Input: part model. Units: mm. Frame: model coordinates. A direction names the side the tool comes from. Coordinates: 2 decimals unless noted, no trailing zeros. Loops run counter-clockwise (first coordinate to the right, second up) from the corner with the lowest first, then second, coordinate; pieces in that order, holes last.
Item 1: Reachability of faces 1 (the flat face through (155, -25, -188)), 2 (the flat face through (-125, -41, -175)), 3 (the flat face through (-95, -25, 187)) from +Z, -Z, +X, -X, +Y, -Y: full face, straight path, thin tool, end or side. Return the list, or none.
Item 2: Section C-C on y = 305. Return loops of the section in (x, z), and give its area (3 significant figures).
Item 3: Pull-direction query (Z, two-part tool) for faces 4 (the flat face through (-3, 83, 200)), 5 (the flat face through (-88, 178, -15)), 6 (the cylindrical face through (139.985, -24.34, -187.675)); classes: released by +Z, released by -Z, zero draft, split by the parting line, or undercut.
Item 4: Section B-B on y = 136.5. Return loops of the section in (x, z).
Item 5: Section D-D on x = 125. Return loops of the section in (y, z).
Item 6: Ray query, line 1 along Z through (x, y) = (-39.5, 155.5); line 2 along X through (y, z) = (158, -143); line 3 along Y through (x, z) = (125, 191). Return the intervals inside material, ascending.
Item 7: Section A-A on z = 0. Return loops of the section in (x, y).
Item 8: Contact query for flat-ended pins moving along their axis: P1, Ø1, axis at x = 151.5, z = -36, coming from the -Y side; P2, Ø23, axis at y = 305, z = 0, coming from the +X side; P3, Ø24, axis at x = -125, y = -25, coming from the +Z side; P4, Ø20, axis at y = -16.5, z = -190.5, coming from the -X side. Output: stop coordinate, or through.
```python
from build123d import *

# Parameters (mm, degrees)
SKETCH1_W            = 450
SKETCH1_H            = 400
BOSS_EXTRUDE1_DEPTH  = 220
SKETCH2_W            = 425
SKETCH2_H            = 375
CUT_EXTRUDE1_DEPTH   = 160
SKETCH3_W            = 280
SKETCH3_H            = 140
CUT_EXTRUDE2_DEPTH   = 12.5
SKETCH4_W            = 30
SKETCH4_H            = 30
BOSS_EXTRUDE2_DEPTH  = 260
SKETCH5_R            = 10
CUT_EXTRUDE3_DEPTH   = 30
SKETCH6_W            = 60
SKETCH6_H            = 25
BOSS_EXTRUDE3_DEPTH  = 50
SKETCH7_R            = 15
CUT_EXTRUDE4_DEPTH   = 25
CUT_EXTRUDE5_START   = -25
SKETCH8_R            = 15
CUT_EXTRUDE5_DEPTH   = 25
CUT_EXTRUDE6_START   = -187.5
CUT_EXTRUDE6_DEPTH   = 375
CUT_EXTRUDE6_2_DEPTH = 172.5
CUT_EXTRUDE6_START_2 = 15
CUT_EXTRUDE6_3_DEPTH = 172.5
SKETCH10_W           = 375
SKETCH10_H           = 197.182681999
CUT_EXTRUDE7_DEPTH   = 12.5


# Read off the part's stored shape, not the designer's step: Cut-Extrude6
with BuildPart() as part:
    # Sketch1 → Boss-Extrude1 (new body)
    with BuildSketch(Plane(origin=(0, 0, 0), x_dir=(1, 0, 0), z_dir=(0, 1, 0))):
        Rectangle(SKETCH1_W, SKETCH1_H)
    extrude(amount=BOSS_EXTRUDE1_DEPTH)

    # Sketch2 → Cut-Extrude1 (cut)
    with BuildSketch(Plane(origin=(0, 220, 0), x_dir=(1, 0, 0), z_dir=(0, 1, 0))):
        Rectangle(SKETCH2_W, SKETCH2_H)
    extrude(amount=-CUT_EXTRUDE1_DEPTH, mode=Mode.SUBTRACT)

    # Sketch3 → Cut-Extrude2 (cut)
    with BuildSketch(Plane(origin=(225, 0, 0), x_dir=(0, 0, -1), z_dir=(1, 0, 0))):
        with Locations((0, 150)):
            Rectangle(SKETCH3_W, SKETCH3_H)
    extrude(amount=-CUT_EXTRUDE2_DEPTH, mode=Mode.SUBTRACT)

    # Sketch4 → Boss-Extrude2 (add)
    with BuildSketch(Plane(origin=(0, 60, 0), x_dir=(1, 0, 0), z_dir=(0, 1, 0))):
        with Locations((-87.5, 0)):
            Rectangle(SKETCH4_W, SKETCH4_H)
    extrude(amount=BOSS_EXTRUDE2_DEPTH)

    # Sketch5 → Cut-Extrude3 (cut)
    with BuildSketch(Plane(origin=(-72.5, 0, 0), x_dir=(0, 0, -1), z_dir=(1, 0, 0))):
        with Locations((0, 305)):
            Circle(SKETCH5_R)
    extrude(amount=-CUT_EXTRUDE3_DEPTH, mode=Mode.SUBTRACT)

    # Sketch6 → Boss-Extrude3 (add)
    with BuildSketch(Plane.XZ):
        with Locations((125, 187.5)):
            Rectangle(SKETCH6_W, SKETCH6_H)
        with Locations((-125, 187.5)):
            Rectangle(SKETCH6_W, SKETCH6_H)
        with Locations((-125, -187.5)):
            Rectangle(SKETCH6_W, SKETCH6_H)
        with Locations((125, -187.5)):
            Rectangle(SKETCH6_W, SKETCH6_H)
    extrude(amount=BOSS_EXTRUDE3_DEPTH)

    # Sketch7 → Cut-Extrude4 (cut)
    with BuildSketch(Plane(origin=(0, 0, -200), x_dir=(-1, 0, 0), z_dir=(0, 0, -1))):
        with Locations((125, -25)):
            Circle(SKETCH7_R)
        with Locations((-125, -25)):
            Circle(SKETCH7_R)
    extrude(amount=-CUT_EXTRUDE4_DEPTH, mode=Mode.SUBTRACT)

    # Sketch8 → Cut-Extrude5 (cut)
    with BuildSketch(Plane.XY.offset(200).offset(CUT_EXTRUDE5_START)):
        with Locations(Location((-125, -25, 0), (0, 0, 180))):
            Circle(SKETCH8_R)
        with Locations(Location((125, -25, 0), (0, 0, 180))):
            Circle(SKETCH8_R)
    extrude(amount=CUT_EXTRUDE5_DEPTH, mode=Mode.SUBTRACT)

    # Cut-Extrude6 outline → Cut-Extrude6 (cut)
    with BuildSketch(Plane.XY.offset(CUT_EXTRUDE6_START)):
        Polygon((-102.5, 60), (-212.5, 60), (-212.5, 22.817318001), (-102.5, 32.441070989), align=None)
        Polygon((212.5, 60), (-72.5, 60), (-72.5, 35.065730895), align=None)
    extrude(amount=CUT_EXTRUDE6_DEPTH, mode=Mode.SUBTRACT)

    # Cut-Extrude6 2 outline → Cut-Extrude6 2 (cut)
    with BuildSketch(Plane.XY.offset(CUT_EXTRUDE6_START)):
        Polygon((-72.5, 60), (-102.5, 60), (-102.5, 32.441070989), (-72.5, 35.065730895), align=None)
    extrude(amount=CUT_EXTRUDE6_2_DEPTH, mode=Mode.SUBTRACT)

    # Cut-Extrude6 3 outline → Cut-Extrude6 3 (cut)
    with BuildSketch(Plane.XY.offset(CUT_EXTRUDE6_START_2)):
        Polygon((-72.5, 60), (-102.5, 60), (-102.5, 32.441070989), (-72.5, 35.065730895), align=None)
    extrude(amount=CUT_EXTRUDE6_3_DEPTH, mode=Mode.SUBTRACT)

    # Sketch10 → Cut-Extrude7 (cut)
    with BuildSketch(Plane(origin=(-212.5, 0, 0), x_dir=(0, 0, -1), z_dir=(1, 0, 0))):
        with Locations((0, 121.408659)):
            Rectangle(SKETCH10_W, SKETCH10_H)
    extrude(amount=-CUT_EXTRUDE7_DEPTH, mode=Mode.SUBTRACT)


solid = part.part
```
Results found:
1. face 1: +Z, -Z, +X, -Y
1. face 2: +X, -X, -Y
1. face 3: +Z, -Z, -Y
2. outline: (-102.5, -15) - (-72.5, -15) - (-72.5, -10) - (-102.5, -10) - close; (-102.5, 10) - (-72.5, 10) - (-72.5, 15) - (-102.5, 15) - close
2. area: 300 mm2
3. face 4: released by +Z
3. face 5: undercut
3. face 6: zero draft
4. outline: (-225, -200) - (225, -200) - (225, -140) - (212.5, -140) - (212.5, -187.5) - (-225, -187.5) - close; (-225, 187.5) - (212.5, 187.5) - (212.5, 140) - (225, 140) - (225, 200) - (-225, 200) - close; (-102.5, -15) - (-72.5, -15) - (-72.5, 15) - (-102.5, 15) - close
5. outline: (-50, -200) - (-40, -200) - (-40, -175) - (-50, -175) - close; (-50, 175) - (-40, 175) - (-40, 200) - (-50, 200) - close; (-10, -200) - (220, -200) - (220, -187.5) - (52.34, -187.5) - (52.34, 187.5) - (220, 187.5) - (220, 200) - (-10, 200) - (-10, 175) - (0, 175) - (0, -175) - (-10, -175) - close
6. line 1: z = -200 to -187.5, 187.5 to 200
6. line 2: x = 212.5 to 225
6. line 3: y = -50 to -40, -10 to 220
7. outline: (-225, 0) - (225, 0) - (225, 80) - (212.5, 80) - (212.5, 60) - (-72.5, 35.07) - (-72.5, 295) - (-102.5, 295) - (-102.5, 32.44) - (-212.5, 22.82) - (-225, 22.82) - close; (-102.5, 315) - (-72.5, 315) - (-72.5, 320) - (-102.5, 320) - close
8. P1: stops at y = 0
8. P2: stops at x = -72.5
8. P3: passes through
8. P4: stops at x = -155
